```python
from build123d import *

# Parameters (mm, degrees)
SKETCH1_W           = 33.65
SKETCH1_H           = 14.7
BOSS_EXTRUDE1_DEPTH = 22.9
SKETCH2_W           = 13.6
SKETCH2_H           = 14.7
BOSS_EXTRUDE2_DEPTH = 18.5
SKETCH3_W           = 6.5
SKETCH3_H           = 2
BOSS_EXTRUDE3_DEPTH = 6.5
SKETCH4_W           = 6.5
SKETCH4_H           = 2
BOSS_EXTRUDE4_DEPTH = 6.5
SKETCH5_R           = 1.996461688
CUT_EXTRUDE1_DEPTH  = 3.75
SKETCH6_R           = 2
CUT_EXTRUDE2_DEPTH  = 3.75
FILLET2_R           = 1
FILLET3_R           = 1


with BuildPart() as part:
    # Sketch1 → Boss-Extrude1 (new body)
    with BuildSketch(Plane(origin=(0, 0, 0), x_dir=(1, 0, 0), z_dir=(0, 1, 0))):
        with Locations((6.48576555, -0.615430622)):
            Rectangle(SKETCH1_W, SKETCH1_H)
    extrude(amount=BOSS_EXTRUDE1_DEPTH)

    # Sketch2 → Boss-Extrude2 (add)
    with BuildSketch(Plane(origin=(0, 22.9, 0), x_dir=(1, 0, 0), z_dir=(0, 1, 0))):
        with Locations((6.48576555, -0.615430622)):
            Rectangle(SKETCH2_W, SKETCH2_H)
    extrude(amount=BOSS_EXTRUDE2_DEPTH)

    # Sketch3 → Boss-Extrude3 (add)
    with BuildSketch(Plane(origin=(0, 22.9, 0), x_dir=(1, 0, 0), z_dir=(0, 1, 0))):
        with Locations((-3.56423445, -6.965430622)):
            Rectangle(SKETCH3_W, SKETCH3_H)
    extrude(amount=BOSS_EXTRUDE3_DEPTH)

    # Sketch4 → Boss-Extrude4 (add)
    with BuildSketch(Plane(origin=(0, 22.9, 0), x_dir=(1, 0, 0), z_dir=(0, 1, 0))):
        with Locations((16.53576555, -6.965430622)):
            Rectangle(SKETCH4_W, SKETCH4_H)
    extrude(amount=BOSS_EXTRUDE4_DEPTH)

    # Sketch5 → Cut-Extrude1 (cut, symmetric)
    with BuildSketch(Plane(origin=(0, 0, 5.965430622), x_dir=(-1, 0, 0), z_dir=(0, 0, -1))):
        with Locations((3.56423445, 26.15)):
            Circle(SKETCH5_R)
    extrude(amount=CUT_EXTRUDE1_DEPTH, both=True, mode=Mode.SUBTRACT)

    # Sketch6 → Cut-Extrude2 (cut, symmetric)
    with BuildSketch(Plane(origin=(0, 0, 5.965430622), x_dir=(-1, 0, 0), z_dir=(0, 0, -1))):
        with Locations((-16.53576555, 26.15)):
            Circle(SKETCH6_R)
    extrude(amount=CUT_EXTRUDE2_DEPTH, both=True, mode=Mode.SUBTRACT)

    # Fillet2
    fillet2_edges = [part.edges().sort_by_distance(p)[0] for p in [
        (23.31076555, 22.9, 0.615430622),
        (-6.81423445, 22.9, 6.965430622),
        (-6.81423445, 29.4, 6.965430622),
        (19.78576555, 22.9, 6.965430622),
        (19.78576555, 29.4, 6.965430622),
        (-10.33923445, 22.9, 0.615430622),
    ]]
    fillet(fillet2_edges, radius=FILLET2_R)

    # Fillet3
    fillet3_edges = [part.edges().sort_by_distance(p)[0] for p in [
        (-4.82673445, 22.9, -6.734569378),
        (-0.31423445, 32.15, -6.734569378),
        (13.28576555, 32.15, -6.734569378),
        (16.03576555, 29.4, 7.965430622),
        (19.78576555, 26.15, 7.965430622),
        (21.54826555, 22.9, 7.965430622),
        (17.79826555, 22.9, -6.734569378),
        (-6.81423445, 26.15, 7.965430622),
        (-8.57673445, 22.9, 7.965430622),
        (-3.06423445, 29.4, 7.965430622),
        (-10.33923445, 10.95, 7.965430622),
        (23.31076555, 10.95, 7.965430622),
        (23.017872331, 22.607106781, 7.965430622),
        (-10.046341231, 22.607106781, 7.965430622),
        (-6.521341231, 29.107106781, 7.965430622),
        (19.492872331, 29.107106781, 7.965430622),
        (-10.33923445, 10.95, -6.734569378),
        (23.31076555, 10.95, -6.734569378),
        (23.017872331, 22.607106781, -6.734569378),
        (-10.046341231, 22.607106781, -6.734569378),
        (20.078658769, 23.192893219, 7.965430622),
        (-7.107127669, 23.192893219, 7.965430622),
    ]]
    fillet(fillet3_edges, radius=FILLET3_R)


solid = part.part
```
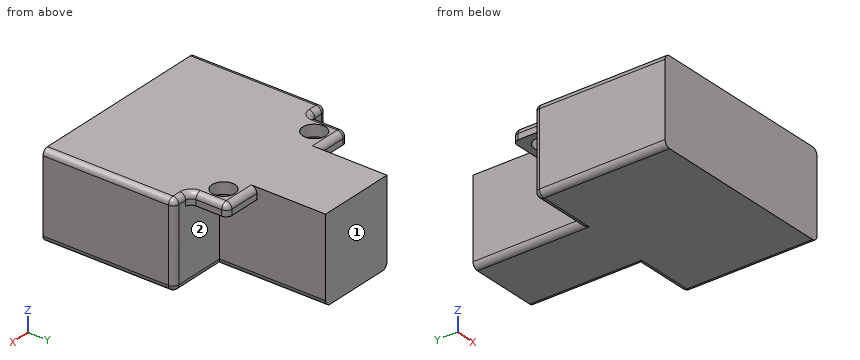
Input: part model. Units: mm. Frame: model coordinates. Face numbers are marked on the shaded views. A direction names the side the tool comes from. Round coordinates to 2 decimals unless told otherwise and drop trailing zeros. Loops run counter-clockwise (first coordinate to the right, second up) from the corner with the lowest first, then second, coordinate; pieces in that order, holes last. Notation, with made-up numbers: (5.25, 63) - (51.25, 63) arc R22 ccw to (51.25, 87) - close; hole circle Ø7 at (-0.75, 72). An arc over 180 degrees is marked (long way). One line per item, written item: value. Start each with the question number.
(1) Access query for the marked faces 1 and 2. Directions: +Z, -Z, +X, -X, +Y, -Y. A direction counts if a zero-diameter tool reaches every point of the face in a straight line with its end or side. Return the directions, or none.
(2) Contact query for flat-ended pins moving along their axis: P1, Ø0.8, axis at x = -1.5, z = 6, coming from the +Y side; P2, Ø0.5, axis at y = 27, z = 6.5, coming from the +X side; P3, Ø5, axis at x = -6, y = 24.5, coming from the -Z side. Output: stop coordinate, or through.
(3) Section A-A, the plane y = 26.15. Return loops of the section in (x, z).
(4) Section B-B, the plane z = -4.25. Return loops of the section in (x, y).
(5) Section C-C, the plane y = 31.5. Return loops of the section in (x, z).
(6) Ray query, line 1 (Y direction, x = 18, z = -1.75); line 2 (X direction, y = 36, z = -1.25); line 3 (Z direction, x = 14.5, y = 28). Return the intervals inside material, ascending. Write a range as [from, to].
Results below:
1. face 1: +Z, -Z, +X, -X, +Y
1. face 2: -Z, +X, +Y
2. P1: y = 29.4
2. P2: x = 19.79
2. P3: z = -6.73
3. outline: (-6.81, 5.97) - (-5.56, 5.97) - (-5.56, 7.97) - (-5.81, 7.97) arc R1 ccw to (-6.81, 6.97) - close; (-1.57, 5.97) - (-0.31, 5.97) - (-0.31, -5.73) arc R1 ccw to (0.69, -6.73) - (12.29, -6.73) arc R1 ccw to (13.29, -5.73) - (13.29, 5.97) - (14.54, 5.97) - (14.54, 7.97) - (-1.57, 7.97) - close; (18.54, 5.97) - (19.79, 5.97) - (19.79, 6.97) arc R1 ccw to (18.79, 7.97) - (18.54, 7.97) - close
4. outline: (-10.34, 0) - (23.31, 0) - (23.31, 21.9) arc R1 ccw to (22.31, 22.9) - (13.29, 22.9) - (13.29, 41.4) - (-0.31, 41.4) - (-0.31, 22.9) - (-9.34, 22.9) arc R1 ccw to (-10.34, 21.9) - close
5. outline: (-0.31, -5.73) arc R1 ccw to (0.69, -6.73) - (12.29, -6.73) arc R1 ccw to (13.29, -5.73) - (13.29, 7.97) - (-0.31, 7.97) - close
6. line 1: [0, 22.9]
6. line 2: [-0.31, 13.29]
6. line 3: [5.97, 7.97]
